Here's how the part is built. I have some questions about the finished solid (model axes, mm). A direction names the side the tool comes from. Coordinates: 2 decimals unless noted, no trailing zeros. Order: outer loops, then holes, each group sorted by start corner. A loop starts at its lowest first (then second) coordinate and runs counter-clockwise, first axis right, second up. Notation, with made-up numbers: (82.25, 72.25) - (141.25, 72.25) arc R9 ccw to (141.25, 84.25) - close; hole circle Ø8 at (12, -12.75). An arc over 180 degrees is marked (long way). Answer as CSV lines item,"result". Start each with the question number.
Item 1: Imagine slicing it at D-D on z = 6.5. List the corners of the cut face in (x, y) for me, and give its area (3 significant figures).
Item 2: We'd pull the mould along Z, two halves only. Please class faces 3 (the face through (0, 3, 13.1)), 4 (the face through (13.93, 2.92, 5.12)), 5 (the face through (17.8, 3, 3)): pulls with the +Z half, pulls with the -Z half, needs draft (parallel to the pull), parting line crosses it, or undercut.
Item 3: Imagine slicing it at B-B on z = 10.3. List the corners of the cut face in (x, y) for me.
Item 4: I need wall thicknesses on line 1 (X direction, y = 1.25, z = 10.3); line 2 (X direction, y = 1.15, z = -1); line 3 (Z direction, x = -8.5, y = 4.05). Which ranges of each line are inside material? Lowest first, please.
Item 5: On a 3-axis mill with a long thin cutter (end or side, diameter ignored), from which of +Z, -Z, +X, -X, +Y, -Y can I reach the whole of each face in a straight line? I mean faces 1 (the face through (-12.2, 1, 0)), 2 (the face through (0, 5.75, 3)). Say none if no direction works.
Item 6: I'm going to push flat-ended pins straight in: pin 1 (2 mm diameter, centred on x = -8.5, z = 10.3, fed in from -Y); pin 2 (3 mm diameter, centred on x = 8.5, z = 10.3, fed in from +Y); pin 3 (1 mm diameter, centred on x = 6, z = 5.5, fed in from -Y). Where does each tip first touch, or does it pass through?
Item 7: Imagine slicing it at C-C on y = 3.25. List the corners of the cut face in (x, z) for me, and give its area (3 significant figures).
Item 8: Imagine slicing it at A-A on x = -15. List the corners of the cut face in (y, z) for me.
from build123d import *

# Parameters (mm, degrees)
BOSS_EXTRUDE1_DEPTH = 7.5
SKETCH8_W           = 35.6
SKETCH8_H           = 5.75
BOSS_EXTRUDE4_DEPTH = 5.6
SKETCH9_R           = 1.35
CUT_EXTRUDE3_DEPTH  = 6.75


with BuildPart() as part:
    # Sketch1 → Boss-Extrude1 (new body, symmetric)
    with BuildSketch(Plane.XY):
        Polygon((-17.8, 5.75), (17.8, 5.75), (17.8, 0), (12.2, 0), (12.2, 2.75), (-12.2, 2.75), (-12.2, 0), (-17.8, 0), align=None)
    extrude(amount=BOSS_EXTRUDE1_DEPTH, both=True)

    # Sketch8 → Boss-Extrude4 (add)
    with BuildSketch(Plane.XY.offset(7.5)):
        with Locations((0, 2.875)):
            Rectangle(SKETCH8_W, SKETCH8_H)
    extrude(amount=BOSS_EXTRUDE4_DEPTH)

    # Sketch9 → Cut-Extrude3 (cut, through all)
    with BuildSketch(Plane(origin=(0, 5.75, 0), x_dir=(1, 0, 0), z_dir=(0, 1, 0))):
        with Locations((-8.5, -10.3)):
            Circle(SKETCH9_R)
        with Locations((-15, -4.3)):
            Circle(SKETCH9_R)
        with Locations((8.5, -10.3)):
            Circle(SKETCH9_R)
        with Locations((15, -4.3)):
            Circle(SKETCH9_R)
    extrude(amount=-CUT_EXTRUDE3_DEPTH, mode=Mode.SUBTRACT)


solid = part.part
Responses:
1,outline,"(-17.8, 0) - (-12.2, 0) - (-12.2, 2.75) - (12.2, 2.75) - (12.2, 0) - (17.8, 0) - (17.8, 5.75) - (-17.8, 5.75) - close"
1,area,"138 mm^2"
2,face 3,"pulls with the +Z half"
2,face 4,"undercut"
2,face 5,"needs draft"
3,outline,"(-17.8, 0) - (-9.85, 0) - (-9.85, 5.75) - (-17.8, 5.75) - close; (-7.15, 0) - (7.15, 0) - (7.15, 5.75) - (-7.15, 5.75) - close; (9.85, 0) - (17.8, 0) - (17.8, 5.75) - (9.85, 5.75) - close"
4,line 1,"x = -17.8 to -9.85, -7.15 to 7.15, 9.85 to 17.8"
4,line 2,"x = -17.8 to -12.2, 12.2 to 17.8"
4,line 3,"z = -7.5 to 8.95, 11.65 to 13.1"
5,face 1,"-Z, -Y"
5,face 2,"+Z, -Z, +X, -X, +Y"
6,pin 1,"passes through"
6,pin 2,"stops at y = 5.75"
6,pin 3,"stops at y = 2.75"
7,outline,"(-17.8, -7.5) - (17.8, -7.5) - (17.8, 13.1) - (-17.8, 13.1) - close; hole circle Ø2.7 at (-15, 4.3); hole circle Ø2.7 at (-8.5, 10.3); hole circle Ø2.7 at (8.5, 10.3); hole circle Ø2.7 at (15, 4.3)"
7,area,"710 mm^2"
8,outline,"(0, -7.5) - (5.75, -7.5) - (5.75, 2.95) - (0, 2.95) - close; (0, 5.65) - (5.75, 5.65) - (5.75, 13.1) - (0, 13.1) - close"
